from build123d import *

# Parameters (mm, degrees)
BOSS_EXTRUDE1_DEPTH = 3
BOSS_EXTRUDE2_START = -0.5
SKETCH1_3_R         = 11
BOSS_EXTRUDE2_DEPTH = 0.5
SKETCH2_R           = 4.1
SKETCH2_R_2         = 1.1
CUT_EXTRUDE1_DEPTH  = 3.5
SKETCH2_3_R         = 2
CUT_EXTRUDE2_DEPTH  = 0.5
CIRPATTERN2_COUNT   = 4
SKETCH1_6_W         = 11
SKETCH1_6_H         = 6
BOSS_EXTRUDE3_DEPTH = 5
SKETCH4_R           = 1.35
CUT_EXTRUDE4_DEPTH  = 8
LPATTERN2_COUNT     = 2
LPATTERN2_PITCH     = 8
LPATTERN2_COL_COUNT = 2
LPATTERN2_COL_PITCH = 8


with BuildPart() as part:
    # Sketch1 → Boss-Extrude1 (new body)
    with BuildSketch(Plane.XY):
        with BuildLine():
            Line((-11, 30), (-11, -30))
            Line((-11, -30), (11, -30))
            Line((11, -30), (11, 30))
            ThreePointArc((11, 30), (0, 41), (-11, 30))
        make_face()
    extrude(amount=BOSS_EXTRUDE1_DEPTH)

    # Sketch1<3> → Boss-Extrude2 (add)
    with BuildSketch(Plane.XY.offset(BOSS_EXTRUDE2_START)):
        with Locations((0, 30)):
            Circle(SKETCH1_3_R)
    extrude(amount=BOSS_EXTRUDE2_DEPTH)

    # Sketch2 → Cut-Extrude1 (cut)
    with BuildSketch(Plane.XY.offset(3)):
        with Locations((0, 30)):
            Circle(SKETCH2_R)
        with Locations((5.656854249, 35.656854249)):
            Circle(SKETCH2_R_2)
    cut_extrude1 = extrude(amount=-CUT_EXTRUDE1_DEPTH, mode=Mode.SUBTRACT)

    # Sketch2<3> → Cut-Extrude2 (cut)
    with BuildSketch(Plane.XY.offset(3)):
        with Locations((5.656854249, 35.656854249)):
            Circle(SKETCH2_3_R)
    cut_extrude2 = extrude(amount=-CUT_EXTRUDE2_DEPTH, mode=Mode.SUBTRACT)

    # CirPattern2: Cut-Extrude1, Cut-Extrude2 ×4 about axis
    cirpattern2_axis = Axis((0, 30, 0), (0, 0, 1))
    add([cut_extrude1.rotate(cirpattern2_axis, i * 360 / CIRPATTERN2_COUNT) for i in range(1, CIRPATTERN2_COUNT)], mode=Mode.SUBTRACT)
    add([cut_extrude2.rotate(cirpattern2_axis, i * 360 / CIRPATTERN2_COUNT) for i in range(1, CIRPATTERN2_COUNT)], mode=Mode.SUBTRACT)

    # Sketch1<6> → Boss-Extrude3 (add)
    with BuildSketch(Plane.XY):
        with Locations((-5.5, -27)):
            Rectangle(SKETCH1_6_W, SKETCH1_6_H)
        with Locations((5.5, -27)):
            Rectangle(SKETCH1_6_W, SKETCH1_6_H)
    extrude(amount=-BOSS_EXTRUDE3_DEPTH)

    # Sketch4 → Cut-Extrude4 (cut)
    with BuildSketch(Plane.XY.offset(3)):
        with Locations((0, -26.6)):
            Circle(SKETCH4_R)
    cut_extrude4 = extrude(amount=-CUT_EXTRUDE4_DEPTH, mode=Mode.SUBTRACT)

    # LPattern2: Cut-Extrude4 ×2
    with Locations(*[(i * LPATTERN2_PITCH, 0, 0) for i in range(1, LPATTERN2_COUNT)]):
        add(cut_extrude4, mode=Mode.SUBTRACT)

    # LPattern2 col: Cut-Extrude4 ×2
    with Locations(*[(-i * LPATTERN2_COL_PITCH, 0, 0) for i in range(1, LPATTERN2_COL_COUNT)]):
        add(cut_extrude4, mode=Mode.SUBTRACT)


solid = part.part
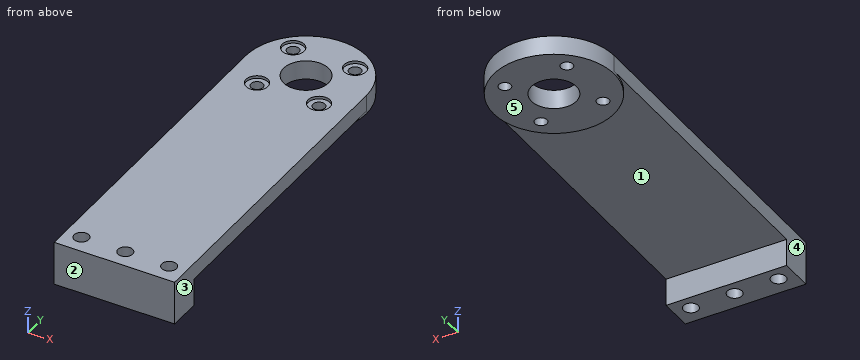
Model file for the job. Use its own axes, mm. Face numbers are marked on the shaded views. A direction names the side the tool comes from. Give positions to 0.01 mm unless a question says otherwise; leave off trailing zeros. Loops run counter-clockwise (first coordinate to the right, second up) from the corner with the lowest first, then second, coordinate; pieces in that order, holes last.
1) Tool access for the marked faces 4 and 5: list every direction of +Z, -Z, +X, -X, +Y, -Y with a clear straight run to the whole face (end or side of a thin tool).
2) Pull direction Y, two halves, no side cores. Call the marked faces 1, 2 and 3: +Y half, -Y half, draft (parallel to the pull), parting line (faces both ways), or undercut.
3) Wall check: line 1 (Y direction, x = 0.25, z = 2.5); line 2 (Y direction, x = 8.25, z = -0.25); line 3 (Z direction, x = -4, y = 38.5). Give the ranges that are in metal, low to high.
4) Saw through at B-B (z = -1.25). Write the cut outline in (x, y).
5) Saw through at D-D (y = -26.6). Write the cut outline in (x, z).
6) Saw through at C-C (y = 27.5). Write the cut outline in (x, z), plus the area to 3 significant figures.
7) Flat gauge pins, fed straight in: pin 1 Ø9.5 at (x, y) = (0, 30) entering from -Z; pin 2 Ø3.5 at (x, y) = (-5.66, 24.34) entering from +Z; pin 3 Ø6 at (x, y) = (4.5, 10.5) entering from -Z. Where does each tip first touch, or does it go through?
8) Saw through at A-A (x = 0). Write the cut outline in (y, z), plus the area to 3 significant figures.
Answer block:
1. face 4: +Z, -Z, -X, +Y, -Y
1. face 5: -Z, +X, -X, +Y
2. face 1: undercut
2. face 2: -Y half
2. face 3: draft
3. line 1: y = -30 to -27.93, -25.27 to 25.91, 34.09 to 41
3. line 2: y = -30 to -27.93, -25.27 to -24, 22.72 to 37.28
3. line 3: z = -0.5 to 3
4. outline: (-11, -30) - (11, -30) - (11, -24) - (-11, -24) - close; hole circle Ø2.7 at (-8, -26.6); hole circle Ø2.7 at (0, -26.6); hole circle Ø2.7 at (8, -26.6)
5. outline: (-11, -5) - (-9.35, -5) - (-9.35, 3) - (-11, 3) - close; (-6.65, -5) - (-1.35, -5) - (-1.35, 3) - (-6.65, 3) - close; (1.35, -5) - (6.65, -5) - (6.65, 3) - (1.35, 3) - close; (9.35, -5) - (11, -5) - (11, 3) - (9.35, 3) - close
6. outline: (-11, 0) - (-10.71, 0) - (-10.71, -0.5) - (-3.25, -0.5) - (-3.25, 3) - (-11, 3) - close; (3.25, -0.5) - (10.71, -0.5) - (10.71, 0) - (11, 0) - (11, 3) - (3.25, 3) - close
6. area: 54.0 mm2
7. pin 1: stops at z = -0.5
7. pin 2: stops at z = 2.5
7. pin 3: stops at z = 0
8. outline: (-30, -5) - (-27.95, -5) - (-27.95, 3) - (-30, 3) - close; (-25.25, -5) - (-24, -5) - (-24, 0) - (19, 0) - (19, -0.5) - (25.9, -0.5) - (25.9, 3) - (-25.25, 3) - close; (34.1, -0.5) - (41, -0.5) - (41, 3) - (34.1, 3) - close
8. area: 204 mm2
